Design review of the part built by this model. Coordinates are the model's own, in mm. Face numbers are marked on the shaded views. A direction names the side the tool comes from. Round coordinates to 2 decimals unless told otherwise and drop trailing zeros. Order: outer loops, then holes, each group sorted by start corner. A loop starts at its lowest first (then second) coordinate and runs counter-clockwise, first axis right, second up. Notation, with made-up numbers: M 11.5,19.5 L 56.5,19.5 A13 cw 56.5,27.5 Z; hole C -34,-13.5 d11. An arc over 180 degrees is marked long. Write item = value, one per line. Start each with the question number.
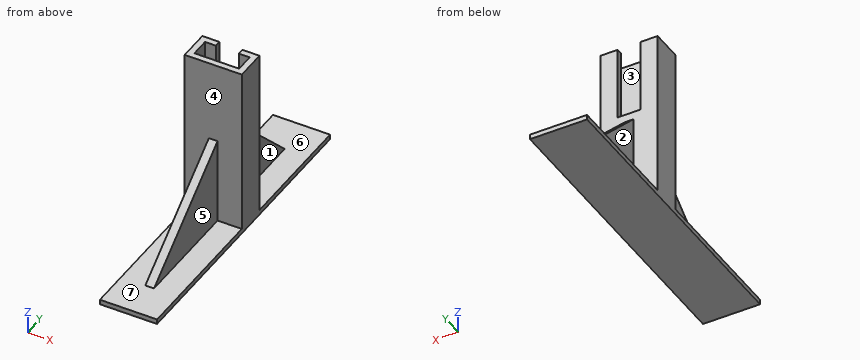
```python
from build123d import *

# Parameters (mm, degrees)
F0_W      = 46
F0_H      = 80
F1_DEPTH  = 25
F4_DEPTH  = 60
F5_DEPTH  = 46
F8_DEPTH  = 3.5
F10_DEPTH = 0.4


with BuildPart() as f1:
    # F0 (on Front) → F1 (new body)
    with BuildSketch(Plane.XZ):
        with Locations((-12.4670048244, -31.5567021806)):
            Rectangle(F0_W, F0_H)
    extrude(amount=F1_DEPTH)

    # F3 (on face) → F4 (join)
    with BuildSketch(Plane.XY.offset(8.4432978194)):
        Polygon((10.5329951756, -25), (10.5329951756, 0), (-3.2170048244, 0), (-3.2170048244, -5), (5.5329951756, -5), (5.5329951756, -20), (-30.4670048244, -20), (-30.4670048244, -5), (-21.7170048244, -5), (-21.7170048244, 0), (-35.4670048244, 0), (-35.4670048244, -25), align=None)
    extrude(amount=F4_DEPTH)

    # F2 (on face) → F5 (join)
    with BuildSketch(Plane(origin=(-35.4670048244, 0, 0), x_dir=(0, -1, 0), z_dir=(-1, 0, 0))):
        Polygon((-100, -71.5567021806), (0, -71.5567021806), (0, -67.5567021806), (-70, -67.5567021806), (-100, -67.5567021806), align=None)
        Polygon((25, -67.5567021806), (25, -71.5567021806), (145, -71.5567021806), (145, -67.5567021806), (115, -67.5567021806), align=None)
    extrude(amount=-F5_DEPTH)

    # F7 (on offset) → F8 (join, symmetric)
    with BuildSketch(Plane(origin=(-12.4670048244, 0, 0), x_dir=(0, -1, 0), z_dir=(-1, 0, 0))):
        Polygon((0, -67.5567021806), (0, 2.4432978194), (-70, -67.5567021806), align=None)
        Polygon((25, 2.4432978194), (25, -67.5567021806), (115, -67.5567021806), align=None)
    extrude(amount=F8_DEPTH, both=True)

    # F10 (add, through all): a face of the model
    f10_faces = [f1.faces().sort_by_distance(p)[0] for p in [
        (-12.4670048244, -11.0375494071, 8.4432978194),
    ]]
    extrude(f10_faces, amount=F10_DEPTH)


solid = f1.part
```
(1) For the marked faces 5, 6 and 7, list the 3-axis set-ups (+Z, -Z, +X, -X, +Y, -Y) from which the entire face can be reached by the end or side of a thin tool; tool diameter is ignored.
(2) Consider section A-A, the plane z = 46. Write out the cut boundary in (x, y), then the cut area to 4 significant figures.
(3) Consider section B-B, the plane x = -27. Write out the cut boundary in (y, z).
(4) For line 1 along Y through (x, z) = (-3, 37); line 2 along Z through (x, y) = (-17.5, -123); line 3 along Y through (x, z) = (-12.5, 58), list the stretches that pass through material, from the lowest coordinate up. Write a range as [from, to].
(5) Consider section C-C, the plane y = 38. Write out the cut boundary in (x, z), then the cut area to 3 significant figures.
(6) Draft analysis for pull direction X (two halves, no side actions). For the marked faces 1, 2, 3 and 4, state which applies: pulls with the +X half, pulls with the -X half, needs draft (parallel to the pull), parting line crosses it, or undercut.
(7) Consider section D-D, the plane y = -68. Write out the cut boundary in (x, z), then the cut area to 3 significant figures.
(8) Insertion check: pin 1 (18 mm diameter, centred on x = -7.5, z = 31.5, fed in from +Y); pin 2 (4.5 mm diameter, centred on x = -27, z = 46.5, fed in from -Y); pin 3 (23 mm diameter, centred on x = -5, z = 7.5, fed in from +Y); pin 4 (10 mm diameter, centred on x = -5.5, y = -27, fed in from +Z). Each pin has a flat end and moves straight along its axis. Give the tip position at first contact, or say it passes through.
Completed:
q1.face_5 = +Z, +X, -Y
q1.face_6 = +Z, +Y
q1.face_7 = +Z, -Y
q2.outline = M -35.47,-25 L 10.53,-25 L 10.53,0 L -3.22,0 L -3.22,-5 L 5.53,-5 L 5.53,-20 L -30.47,-20 L -30.47,-5 L -21.72,-5 L -21.72,0 L -35.47,0 Z
q2.area = 517.5 mm2
q3.outline = M -145,-71.56 L 100,-71.56 L 100,-67.56 L 0,-67.56 L 0,68.44 L -5,68.44 L -5,8.84 L -20,8.84 L -20,68.44 L -25,68.44 L -25,-67.56 L -145,-67.56 Z
q4.line_1 = [-25, -20], [-5, 0]
q4.line_2 = [-71.56, -67.56]
q4.line_3 = [-25, -20]
q5.outline = M -35.47,-71.56 L 10.53,-71.56 L 10.53,-67.56 L -8.97,-67.56 L -8.97,-35.56 L -15.97,-35.56 L -15.97,-67.56 L -35.47,-67.56 Z
q5.area = 408 mm2
q6.face_1 = pulls with the +X half
q6.face_2 = pulls with the -X half
q6.face_3 = undercut
q6.face_4 = needs draft
q7.outline = M -35.47,-71.56 L 10.53,-71.56 L 10.53,-67.56 L -8.97,-67.56 L -8.97,-31 L -15.97,-31 L -15.97,-67.56 L -35.47,-67.56 Z
q7.area = 440 mm2
q8.pin_1 = 0
q8.pin_2 = -25
q8.pin_3 = 5.74
q8.pin_4 = 68.44
